The listing builds one solid part. Answer for the finished solid, in the listing's coordinates (mm). A direction names the side the tool comes from. Round coordinates to 2 decimals unless told otherwise and drop trailing zeros. Order: outer loops, then holes, each group sorted by start corner. A loop starts at its lowest first (then second) coordinate and runs counter-clockwise, first axis right, second up. Notation, with made-up numbers: (-1.75, -14) - (38.25, -14) arc R19 ccw to (38.25, 22) - close; hole circle Ø1 at (-14.75, -27.75). An arc over 180 degrees is marked (long way). Use CSV: the item, a comma, the result in double quotes. Start each with the question number.
Item 1: Determine the mould class of faces 4 (the cylindrical face through (23.846, 7.509, 36.975)), 5 (the cylindrical face through (-2.17, -9.76, 34.51)), 6 (the flat face through (0, 0, 150)), 7 (the flat face through (10, -5, 70)) for opening direction Y: +Y half, -Y half, draft (parallel to the pull), parting line (faces both ways), or undercut.
Item 2: Flat-ended cylindrical pins translate along their axes: P1, Ø8, axis at y = -18, z = 60, coming from the +X side; P2, Ø10, axis at y = 7, z = 133.5, coming from the -X side; P3, Ø6, axis at x = 2.5, y = 17.5, coming from the -Z side. Find the tip coordinate at first contact, or state that the pin passes through.
Item 3: For faces 1 (the flat face through (0, 0, 0)), 2 (the cylindrical face through (-0.867, -3.905, 111.975)), 3 (the cylindrical face through (22.4, 7.1, 34.5)), determine the directions among +Z, -Z, +X, -X, +Y, -Y from which every point of the face is accessible in a straight line to the end or side of a thin tool.
Item 4: Find section A-A, the plane z = 21. Give the vertices of the cut face in (x, y), plus the area to 3 significant figures.
Item 5: Find section B-B, the plane y = 0. Give the vertices of the cut face in (x, z).
Item 6: Straight lines are drawn through the part: line 1 along Y through (x, z) = (0, 21); line 2 along X through (y, z) = (-6.5, 61.5); line 3 along Y through (x, z) = (-9, 15). For each, find the intervals that lie inside material, in ascending order. Write a range as [from, to].
Item 7: Find section D-D, the plane z = 138. Give the vertices of the cut face in (x, y), plus the area to 3 significant figures.
```python
from build123d import *

# Parameters (mm, degrees)
F0_R     = 25
F0_R_2   = 23.5
F1_DEPTH = 70
F2_R     = 25
F3_DEPTH = 5
F4_R     = 4
F5_DEPTH = 75
F0_R_3   = 10
F6_DEPTH = 75


with BuildPart() as f1:
    # F0 (on Top) → F1 (new body)
    with BuildSketch(Plane.XY):
        Circle(F0_R)
        Circle(F0_R_2, mode=Mode.SUBTRACT)
    extrude(amount=F1_DEPTH)

    # F2 (on face) → F3 (join)
    with BuildSketch(Plane.XY.offset(70)):
        Circle(F2_R)
    extrude(amount=F3_DEPTH)

    # F4 (on face) → F5 (join)
    with BuildSketch(Plane.XY.offset(75)):
        Circle(F4_R)
    extrude(amount=F5_DEPTH)

    # F0 (on Top) → F6 (join)
    with BuildSketch(Plane.XY):
        Circle(F0_R_3)
    extrude(amount=F6_DEPTH)


solid = f1.part
```
Worked out:
1,face 4,"parting line"
1,face 5,"undercut"
1,face 6,"draft"
1,face 7,"undercut"
2,P1,"stops at x = 20.71"
2,P2,"stops at x = -3.46"
2,P3,"stops at z = 70"
3,face 1,"-Z, +X, -X, +Y, -Y"
3,face 2,"+Z"
3,face 3,"-Z"
4,outline,"circle Ø50 at (0, 0); circle Ø20 at (0, 0); hole circle Ø47 at (0, 0)"
4,area,"543 mm²"
5,outline,"(-25, 0) - (-23.5, 0) - (-23.5, 70) - (-10, 70) - (-10, 0) - (10, 0) - (10, 70) - (23.5, 70) - (23.5, 0) - (25, 0) - (25, 75) - (4, 75) - (4, 150) - (-4, 150) - (-4, 75) - (-25, 75) - close"
6,line 1,"y = [-25, -23.5], [-10, 10], [23.5, 25]"
6,line 2,"x = [-24.14, -22.58], [-7.6, 7.6], [22.58, 24.14]"
6,line 3,"y = [-23.32, -21.71], [-4.36, 4.36], [21.71, 23.32]"
7,outline,"circle Ø8 at (0, 0)"
7,area,"50.3 mm²"
